Design review of the part built by this model. Coordinates are the model's own, in mm. A direction names the side the tool comes from. Give positions to 0.01 mm unless a question says otherwise; leave off trailing zeros. Loops run counter-clockwise (first coordinate to the right, second up) from the corner with the lowest first, then second, coordinate; pieces in that order, holes last. Notation, with made-up numbers: (-10.5, 86) - (4.5, 86) arc R15 cw to (4.5, 101) - close; hole circle Ø7 at (32, 14.25). An arc over 180 degrees is marked (long way). Write each question's results on one line, items separated by ' | '.
```python
from build123d import *

# Parameters (mm, degrees)
SKETCH1_R           = 31.75
SKETCH1_R_2         = 3.175
SKETCH1_R_3         = 15.875
SKETCH1_R_4         = 9.5504
BOSS_EXTRUDE1_DEPTH = 3.175
SKETCH2_R           = 3.175
CUT_EXTRUDE1_DEPTH  = 1.5875


with BuildPart() as part:
    # Sketch1 → Boss-Extrude1 (new body)
    # profile 1 of 2: a face of its own
    with BuildSketch(Plane.XY.offset(191.201675)):
        with Locations((0, 762.756140976)):
            Circle(SKETCH1_R)
        with Locations((-21.997045256, 775.456140976)):
            Circle(SKETCH1_R_2, mode=Mode.SUBTRACT)
        with Locations((-21.997045256, 750.056140976)):
            Circle(SKETCH1_R_2, mode=Mode.SUBTRACT)
        with Locations((0, 737.356140976)):
            Circle(SKETCH1_R_2, mode=Mode.SUBTRACT)
        with Locations((21.997045256, 750.056140976)):
            Circle(SKETCH1_R_2, mode=Mode.SUBTRACT)
        with Locations((21.997045256, 775.456140976)):
            Circle(SKETCH1_R_2, mode=Mode.SUBTRACT)
        with Locations((0, 788.156140976)):
            Circle(SKETCH1_R_2, mode=Mode.SUBTRACT)
        with Locations((0, 762.756140976)):
            Circle(SKETCH1_R_3, mode=Mode.SUBTRACT)
    # profile 2 of 2: a face of its own
    with BuildSketch(Plane.XY.offset(191.201675)):
        with Locations((0, 762.756140976)):
            Circle(SKETCH1_R_3)
        with Locations((0, 762.756140976)):
            Circle(SKETCH1_R_4, mode=Mode.SUBTRACT)
    extrude(amount=BOSS_EXTRUDE1_DEPTH)

    # Sketch2 → Cut-Extrude1 (cut)
    with BuildSketch(Plane.XY.offset(194.376675)):
        with Locations((-14.2875, 762.756140976)):
            Circle(SKETCH2_R)
        with Locations((14.2875, 762.756140976)):
            Circle(SKETCH2_R)
    extrude(amount=-CUT_EXTRUDE1_DEPTH, mode=Mode.SUBTRACT)


solid = part.part
```
Item 1: We need section A-A on x = 0. Give the boundary of the cut face in (y, z), then the cut area to 3 significant figures.
Output values:
outline: (731.01, 191.2) - (734.18, 191.2) - (734.18, 194.38) - (731.01, 194.38) - close; (740.53, 191.2) - (753.21, 191.2) - (753.21, 194.38) - (740.53, 194.38) - close; (772.31, 191.2) - (784.98, 191.2) - (784.98, 194.38) - (772.31, 194.38) - close; (791.33, 191.2) - (794.51, 191.2) - (794.51, 194.38) - (791.33, 194.38) - close | area: 101 mm²
Item 2: Tool access review of faces 1 (the face through (-24.5, 748.1, 192.8)), 2 (the face through (-14, 763, 192.789)): name each direction out of +Z, -Z, +X, -X, +Y, -Y from which nothing blocks a thin tool from reaching the whole face with its end or side.
Output values:
face 1: +Z, -Z | face 2: +Z
Item 3: Wall thickness on probe 1 along Y at (x, z) = (0, 191.95); probe 2 along X at (y, z) = (747.5, 191.5); probe 3 along Y at (x, z) = (-22.5, 193.9): over which ranges is each line inside the solid? List them lowest first.
Output values:
probe 1: y = 731.01 to 734.18, 740.53 to 753.21, 772.31 to 784.98, 791.33 to 794.51 | probe 2: x = -27.84 to -23.88, -20.11 to 20.11, 23.88 to 27.84 | probe 3: y = 740.35 to 746.92, 753.19 to 772.32, 778.59 to 785.16
Item 4: We need section D-D on x = -21. Give the boundary of the cut face in (y, z).
Output values:
outline: (738.94, 191.2) - (747.04, 191.2) - (747.04, 194.38) - (738.94, 194.38) - close; (753.07, 191.2) - (772.44, 191.2) - (772.44, 194.38) - (753.07, 194.38) - close; (778.47, 191.2) - (786.57, 191.2) - (786.57, 194.38) - (778.47, 194.38) - close
Item 5: We need section B-B on y = 769.5. Give the boundary of the cut face in (x, z), then the cut area to 3 significant figures.
Output values:
outline: (-31.03, 191.2) - (-6.76, 191.2) - (-6.76, 194.38) - (-31.03, 194.38) - close; (6.76, 191.2) - (31.03, 191.2) - (31.03, 194.38) - (6.76, 194.38) - close | area: 154 mm²
Item 6: We need section C-C on z = 193.5. Give the number of separate pieces and of enclosed holes in the cut face, then the cut area to 3 significant figures.
Output values:
separate pieces: 1 | enclosed holes: 9 | area: 2,630 mm²
Item 7: Clearance check with flat-ended pins moving along their axes: P1, Ø1.9, axis at x = 14.5, y = 764, coming from the +Z side; P2, Ø1.5, axis at y = 787, z = 193.5, coming from the +X side. State where each tip first meets the part, or that it passes through.
Output values:
P1: stops at z = 192.79 | P2: stops at x = 21.36
Item 8: Draft analysis for pull direction X (two halves, no side actions). For faces 3 (the face through (-2.07, 753.433, 192.767)), 4 (the face through (-4.133, 794.236, 192.767)), 5 (the face through (-22.41, 778.604, 192.767)), 6 (the face through (7, 770, 194.377)), state which applies: +X half, -X half, draft (parallel to the pull), parting line (faces both ways), or undercut.
Output values:
face 3: undercut | face 4: parting line | face 5: undercut | face 6: draft
